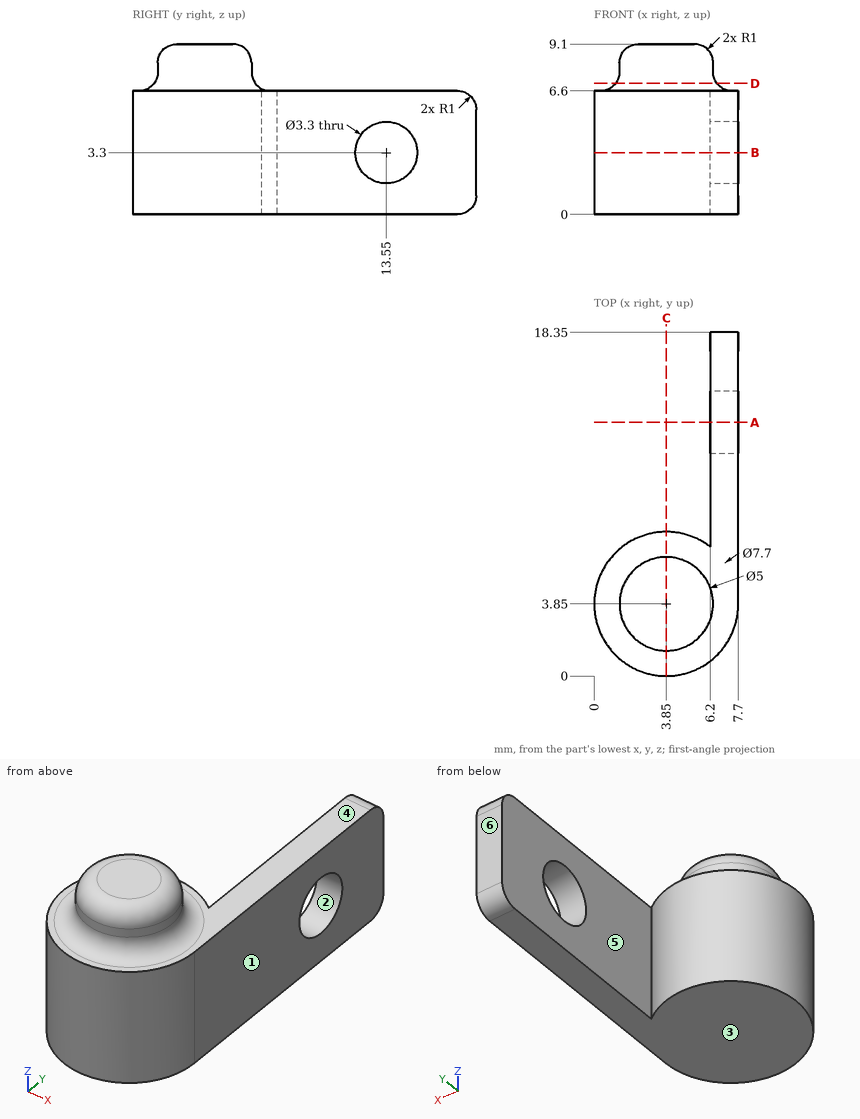
Could you check a few things on this drawing? It's one solid part, dimensions in mm from its lowest x, y, z. A direction names the side the tool comes from. Give positions to 0.01 mm unless a question says otherwise; leave off trailing zeros. Order: outer loops, then holes, each group sorted by start corner. A loop starts at its lowest first (then second) coordinate and runs counter-clockwise, first axis right, second up. Notation, with made-up numbers: (3, -32) -> (46, -32) arc R24 ccw to (46, 1) -> close; hole circle Ø5 at (-13.75, 36.5). An arc over 180 degrees is marked (long way). Answer in a Markdown table with one row per item. Add a question column.
Item 1: Imagine slicing it at B-B (z = 3.3). List the corners of the cut face in (x, y) for me, and give its area (3 significant figures).
Item 2: Please list where these lines run through material, in increasing order: probe 1 along Z at (x, y) = (7.3, 13.55); probe 2 along X at (y, z) = (8.5, 2.5); probe 3 along X at (y, z) = (2.25, 6).
Item 3: For the marked faces 4, 5 and 6, which set-ups out of +Z, -Z, +X, -X, +Y, -Y let a thin tool reach every point of the face, with its end or its side?
Item 4: I'm going to push flat-ended pins straight in: P1, Ø1.5, axis at x = 6, y = 9.5, coming from the +Z side; P2, Ø4, axis at x = 6, z = 7.5, coming from the -Y side; P3, Ø2.5, axis at x = 3.5, y = 9.5, coming from the +Z side; P4, Ø4, axis at x = 5.5, y = 11, coming from the -Z side. Where does each tip first touch, or does it pass through?
Item 5: Imagine slicing it at D-D (z = 7). List the corners of the cut face in (x, y) for me.
Item 6: We'd pull the mould along Z, two halves only. Please class the marked faces 1, 2 and 3: pulls with the +Z half, pulls with the -Z half, needs draft (parallel to the pull), parting line crosses it, or undercut.
Item 7: Imagine slicing it at C-C (x = 3.85). List the corners of the cut face in (y, z) for me, and give its area (3 significant figures).
Item 8: Imagine slicing it at A-A (y = 13.55). List the corners of the cut face in (x, z) for me, and give its area (3 significant figures).
Result:
| question | item | result |
|---|---|---|
| 1 | outline | (6.2, 6.9) arc R3.85 ccw (long way) to (7.7, 3.85) -> (7.7, 11.9) -> (6.2, 11.9) -> close; (6.2, 15.2) -> (7.7, 15.2) -> (7.7, 18.35) -> (6.2, 18.35) -> close |
| 1 | area | 60.2 mm2 |
| 2 | probe 1 | 0 to 1.65, 4.95 to 6.6 |
| 2 | probe 2 | 6.2 to 7.7 |
| 2 | probe 3 | 0.35 to 7.35 |
| 3 | face 4 | +Z |
| 3 | face 5 | +Z, -Z, +Y |
| 3 | face 6 | +Z, -Z, +X, -X, +Y |
| 4 | P1 | z = 6.6 |
| 4 | P2 | y = 0.02 |
| 4 | P3 | through |
| 4 | P4 | z = 0 |
| 5 | outline | circle Ø5.4 at (3.85, 3.85) |
| 6 | face 1 | needs draft |
| 6 | face 2 | undercut |
| 6 | face 3 | pulls with the -Z half |
| 7 | outline | (0, 0) -> (7.7, 0) -> (7.7, 6.6) -> (7.35, 6.6) arc R1 cw to (6.35, 7.6) -> (6.35, 8.1) arc R1 ccw to (5.35, 9.1) -> (2.35, 9.1) arc R1 ccw to (1.35, 8.1) -> (1.35, 7.6) arc R1 cw to (0.35, 6.6) -> (0, 6.6) -> close |
| 7 | area | 63.3 mm2 |
| 8 | outline | (6.2, 0) -> (7.7, 0) -> (7.7, 1.65) -> (6.2, 1.65) -> close; (6.2, 4.95) -> (7.7, 4.95) -> (7.7, 6.6) -> (6.2, 6.6) -> close |
| 8 | area | 4.95 mm2 |
